Autodesk Inventor part; units mm, degrees
ref_plane "YZ Plane" through (0, 0, 0) normal (1, 0, 0) x (0, 1, 0)
ref_plane "XZ Plane" through (0, 0, 0) normal (0, 1, 0) x (-1, 0, 0)
ref_plane "XY Plane" through (0, 0, 0) normal (0, 0, 1) x (1, 0, 0)
sketch "Sketch1" plane through (0, 0, 0) normal (0, 0, 1) x (1, 0, 0)
  line L0 (12.7, -31.75) -> (15.5956, -31.75)
  line L1 (15.5956, -31.75) -> (34.6456, -31.75)
  line L2 (34.6456, -31.75) -> (34.6456, -12.7)
  line L3 (34.6456, -12.7) -> (31.75, -12.7)
  line L4 (31.75, -12.7) -> (31.75, 12.7)
  line L5 (31.75, 12.7) -> (34.6456, 12.7)
  line L6 (34.6456, 12.7) -> (34.6456, 31.75)
  line L7 (34.6456, 31.75) -> (15.5956, 31.75)
  line L8 (15.5956, 31.75) -> (12.7, 31.75)
  line L9 (12.7, 31.75) -> (12.7, 34.6456)
  line L10 (12.7, 34.6456) -> (-12.7, 34.6456)
  line L11 (-12.7, 34.6456) -> (-12.7, 31.75)
  line L12 (-12.7, 31.75) -> (-15.5956, 31.75)
  line L13 (-15.5956, 31.75) -> (-34.6456, 31.75)
  line L14 (-34.6456, 31.75) -> (-34.6456, 12.7)
  line L15 (-34.6456, 12.7) -> (-31.75, 12.7)
  line L16 (-31.75, 12.7) -> (-31.75, -12.7)
  line L17 (-31.75, -12.7) -> (-34.6456, -12.7)
  line L18 (-34.6456, -12.7) -> (-34.6456, -31.75)
  line L19 (-34.6456, -31.75) -> (-15.5956, -31.75)
  line L20 (-15.5956, -31.75) -> (-12.7, -31.75)
  line L21 (-12.7, -31.75) -> (-12.7, -34.6456)
  line L22 (-12.7, -34.6456) -> (12.7, -34.6456)
  line L23 (12.7, -34.6456) -> (12.7, -31.75)
  point P0 (0, 0)
extrude "Extrusion1" add sketch "Sketch1" along normal blind 2.8956
properties part number "outside_box_left_right" material "Polycarbonate, Clear"
Design review of the part built by this model. Coordinates are the model's own, in mm. A direction names the side the tool comes from. Coordinates: 2 decimals unless noted, no trailing zeros. Loops run counter-clockwise (first coordinate to the right, second up) from the corner with the lowest first, then second, coordinate; pieces in that order, holes last. Notation, with made-up numbers: M 51.5,5.25 L 70.5,5.25 A9 cw 70.5,10.25 Z; hole C -2.75,88 d4. An arc over 180 degrees is marked long. Answer as CSV lines item,"result".
Item 1: Machinability: for faces 4 (the face through (24, -31.75, 1)), 5 (the face through (-12.7, 33, 1)), 6 (the face through (-12.7, -33, 1)), 7 (the face through (31.75, 0, 1)), 8 (the face through (-33, 12.7, 1)), which of the approach directions +Z, -Z, +X, -X, +Y, -Y give a long, thin tool a straight path to every point of the face, cutting with its end or side? Answer none if there is none.
Answer list:
face 4,"+Z, -Z, +X, -Y"
face 5,"+Z, -Z, -X, +Y"
face 6,"+Z, -Z, -X, -Y"
face 7,"+Z, -Z, +X"
face 8,"+Z, -Z, -X"
Item 2: For P1, Ø1.4, axis at x = -19, z = 1, coming from the +Y side; P2, Ø0.9, axis at x = -34, z = 1.5, coming from the -Y side, all flat-tipped, find the tip position at first contact; note any pin that passes through.
Answer list:
P1,"y = 31.75"
P2,"y = -31.75"
Item 3: Add section A-A on z = 2.4. State the section outline as (x, y) points.
Answer list:
outline,"M -34.65,-31.75 L -12.7,-31.75 L -12.7,-34.65 L 12.7,-34.65 L 12.7,-31.75 L 34.65,-31.75 L 34.65,-12.7 L 31.75,-12.7 L 31.75,12.7 L 34.65,12.7 L 34.65,31.75 L 12.7,31.75 L 12.7,34.65 L -12.7,34.65 L -12.7,31.75 L -34.65,31.75 L -34.65,12.7 L -31.75,12.7 L -31.75,-12.7 L -34.65,-12.7 Z"
Item 4: Add section B-B on y = -11. State the section outline as (x, z) points.
Answer list:
outline,"M -31.75,0 L 31.75,0 L 31.75,2.9 L -31.75,2.9 Z"
Item 5: The part is to be moulded in two halves that separate along Y. For faces 1 (the face through (-31.75, 0, 1)), 2 (the face through (-24, -31.75, 1)), 3 (the face through (12.7, -33, 1)), say which applies: pulls with the +Y half, pulls with the -Y half, needs draft (parallel to the pull), parting line crosses it, or undercut.
Answer list:
face 1,"undercut"
face 2,"pulls with the -Y half"
face 3,"needs draft"
Item 6: For probe 1 along Y at (x, z) = (32.5, 1); probe 2 along Y at (x, z) = (20, 0.7), list the stretches that pass through material, from the lowest coordinate up.
Answer list:
probe 1,"-31.75 to -12.7, 12.7 to 31.75"
probe 2,"-31.75 to 31.75"
